```python
from build123d import *

# Parameters (mm, degrees)
ESQUISSE1_R             = 6
BOSS_EXTRU_2_DEPTH      = 10
CONG_2_R                = 1
ESQUISSE5_R             = 4
ENL_V_MAT_EXTRU_2_DEPTH = 14.114877094
COQUE5_T                = -0.2
BOSS_EXTRU_5_REACH      = 14.963


with BuildPart() as part:
    # Esquisse1 → Boss.-Extru.2 (new body)
    with BuildSketch(Plane.XY):
        Circle(ESQUISSE1_R)
    extrude(amount=BOSS_EXTRU_2_DEPTH)

    # Congé2
    cong_2_edges = [part.edges().sort_by_distance(p)[0] for p in [
        (-6, 0, 0),
        (-6, 0, 10),
    ]]
    fillet(cong_2_edges, radius=CONG_2_R)

    # Esquisse5 → Enlèv. mat.-Extru.2 (cut, through all)
    with BuildSketch(Plane.XY.offset(10)):
        Circle(ESQUISSE5_R)
    extrude(amount=-ENL_V_MAT_EXTRU_2_DEPTH, mode=Mode.SUBTRACT)

    # Coque5
    coque5_openings = [part.faces().sort_by_distance(p)[0] for p in [
        (-4, 0, 5),
    ]]
    offset(amount=COQUE5_T, openings=coque5_openings, kind=Kind.INTERSECTION)

    # Esquisse12 → Boss.-Extru.5 (add, up to next)
    with BuildSketch(Plane.XY.offset(0.2), mode=Mode.PRIVATE) as boss_extru_5_sk1:
        with BuildLine():
            ThreePointArc((-4.089017574, 1.521224294), (-4.253433845, 0.970818519), (-4.344112019, 0.403582504))
            ThreePointArc((-4.344112019, 0.403582504), (-4.932642925, 0), (-4.344112019, -0.403582504))
            ThreePointArc((-4.344112019, -0.403582504), (-4.253433845, -0.970818519), (-4.089017574, -1.521224294))
            ThreePointArc((-4.089017574, -1.521224294), (-4.444157712, -2.140193556), (-3.738801802, -2.248454838))
            ThreePointArc((-3.738801802, -2.248454838), (-3.410989107, -2.720173043), (-3.02404305, -3.144733964))
            ThreePointArc((-3.02404305, -3.144733964), (-3.07545256, -3.85649553), (-2.392976034, -3.647993115))
            ThreePointArc((-2.392976034, -3.647993115), (-1.892956143, -3.930763935), (-1.360119712, -4.145390505))
            ThreePointArc((-1.360119712, -4.145390505), (-1.097616311, -4.808971268), (-0.573192015, -4.325001617))
            ThreePointArc((-0.573192015, -4.325001617), (0, -4.362818822), (0.573192015, -4.325001617))
            ThreePointArc((0.573192015, -4.325001617), (1.097616311, -4.808971268), (1.360119712, -4.145390505))
            ThreePointArc((1.360119712, -4.145390505), (1.892956143, -3.930763935), (2.392976034, -3.647993115))
            ThreePointArc((2.392976034, -3.647993115), (3.07545256, -3.85649553), (3.02404305, -3.144733964))
            ThreePointArc((3.02404305, -3.144733964), (3.410989107, -2.720173043), (3.738801802, -2.248454838))
            ThreePointArc((3.738801802, -2.248454838), (4.444157712, -2.140193556), (4.089017574, -1.521224294))
            ThreePointArc((4.089017574, -1.521224294), (4.253433845, -0.970818519), (4.344112019, -0.403582504))
            ThreePointArc((4.344112019, -0.403582504), (4.932642925, 0), (4.344112019, 0.403582504))
            ThreePointArc((4.344112019, 0.403582504), (4.253433845, 0.970818519), (4.089017574, 1.521224294))
            ThreePointArc((4.089017574, 1.521224294), (4.444157712, 2.140193556), (3.738801802, 2.248454838))
            ThreePointArc((3.738801802, 2.248454838), (3.410989107, 2.720173043), (3.02404305, 3.144733964))
            ThreePointArc((3.02404305, 3.144733964), (3.07545256, 3.85649553), (2.392976034, 3.647993115))
            ThreePointArc((2.392976034, 3.647993115), (1.892956143, 3.930763935), (1.360119712, 4.145390505))
            ThreePointArc((1.360119712, 4.145390505), (1.097616311, 4.808971268), (0.573192015, 4.325001617))
            ThreePointArc((0.573192015, 4.325001617), (0, 4.362818822), (-0.573192015, 4.325001617))
            ThreePointArc((-0.573192015, 4.325001617), (-1.097616311, 4.808971268), (-1.360119712, 4.145390505))
            ThreePointArc((-1.360119712, 4.145390505), (-1.892956143, 3.930763935), (-2.392976034, 3.647993115))
            ThreePointArc((-2.392976034, 3.647993115), (-3.07545256, 3.85649553), (-3.02404305, 3.144733964))
            ThreePointArc((-3.02404305, 3.144733964), (-3.410989107, 2.720173043), (-3.738801802, 2.248454838))
            ThreePointArc((-3.738801802, 2.248454838), (-4.444157712, 2.140193556), (-4.089017574, 1.521224294))
        make_face()
        with BuildLine():
            ThreePointArc((-3.940916918, 1.53497163), (-4.123260956, 0.941107406), (-4.216642684, 0.326938116))
            ThreePointArc((-4.216642684, 0.326938116), (-4.067357075, 0), (-4.216642684, -0.326938116))
            ThreePointArc((-4.216642684, -0.326938116), (-4.123260956, -0.941107406), (-3.940916918, -1.53497163))
            ThreePointArc((-3.940916918, -1.53497163), (-3.664562099, -1.764760096), (-3.657210653, -2.124093759))
            ThreePointArc((-3.657210653, -2.124093759), (-3.306598555, -2.636924355), (-2.884644224, -3.092861419))
            ThreePointArc((-2.884644224, -3.092861419), (-2.535955657, -3.179987812), (-2.373423199, -3.500546582))
            ThreePointArc((-2.373423199, -3.500546582), (-1.835023758, -3.810466096), (-1.257032364, -4.038172073))
            ThreePointArc((-1.257032364, -4.038172073), (-0.905072095, -3.965379941), (-0.619550173, -4.183673224))
            ThreePointArc((-0.619550173, -4.183673224), (0, -4.229298294), (0.619550173, -4.183673224))
            ThreePointArc((0.619550173, -4.183673224), (0.905072095, -3.965379941), (1.257032364, -4.038172073))
            ThreePointArc((1.257032364, -4.038172073), (1.835023758, -3.810466096), (2.373423199, -3.500546582))
            ThreePointArc((2.373423199, -3.500546582), (2.535955657, -3.179987812), (2.884644224, -3.092861419))
            ThreePointArc((2.884644224, -3.092861419), (3.306598555, -2.636924355), (3.657210653, -2.124093759))
            ThreePointArc((3.657210653, -2.124093759), (3.664562099, -1.764760096), (3.940916918, -1.53497163))
            ThreePointArc((3.940916918, -1.53497163), (4.123260956, -0.941107406), (4.216642684, -0.326938116))
            ThreePointArc((4.216642684, -0.326938116), (4.067357075, 0), (4.216642684, 0.326938116))
            ThreePointArc((4.216642684, 0.326938116), (4.123260956, 0.941107406), (3.940916918, 1.53497163))
            ThreePointArc((3.940916918, 1.53497163), (3.664562099, 1.764760096), (3.657210653, 2.124093759))
            ThreePointArc((3.657210653, 2.124093759), (3.306598555, 2.636924355), (2.884644224, 3.092861419))
            ThreePointArc((2.884644224, 3.092861419), (2.535955657, 3.179987812), (2.373423199, 3.500546582))
            ThreePointArc((2.373423199, 3.500546582), (1.835023758, 3.810466096), (1.257032364, 4.038172073))
            ThreePointArc((1.257032364, 4.038172073), (0.905072095, 3.965379941), (0.619550173, 4.183673224))
            ThreePointArc((0.619550173, 4.183673224), (0, 4.229298294), (-0.619550173, 4.183673224))
            ThreePointArc((-0.619550173, 4.183673224), (-0.905072095, 3.965379941), (-1.257032364, 4.038172073))
            ThreePointArc((-1.257032364, 4.038172073), (-1.835023758, 3.810466096), (-2.373423199, 3.500546582))
            ThreePointArc((-2.373423199, 3.500546582), (-2.535955657, 3.179987812), (-2.884644224, 3.092861419))
            ThreePointArc((-2.884644224, 3.092861419), (-3.306598555, 2.636924355), (-3.657210653, 2.124093759))
            ThreePointArc((-3.657210653, 2.124093759), (-3.664562099, 1.764760096), (-3.940916918, 1.53497163))
        make_face(mode=Mode.SUBTRACT)
    boss_extru_5_tool1 = extrude(boss_extru_5_sk1.sketch, amount=BOSS_EXTRU_5_REACH, mode=Mode.PRIVATE) - part.part
    add(boss_extru_5_tool1.solids().sort_by_distance((-3.400205, 2.711573, 0.2))[0])


solid = part.part
```
Geometry check sheet. Reference: the model listing, model coordinates, mm. Coordinates: 2 decimals unless noted, no trailing zeros. Answer as a JSON object with one key per item and string values. Group by question number.
Item 1: Depth check by flat-ended pin: pin 1 Ø6.5 at (x, y) = (0, 0) entering from +Z (1 decimal); pin 2 Ø6 at (x, y) = (-2.5, -4.5) entering from -Z; pin 3 Ø5 at (x, z) = (-3.5, 5) entering from +Y; pin 4 Ø1.5 at (x, z) = (-3, 4) entering from +Y. Enter the tip coordinate at first touch or a pass-through.
Item 2: Scan lines: probe 1 along X at (y, z) = (3.25, 4.5); probe 2 along Z at (x, y) = (3.75, 3); probe 3 along Y at (x, z) = (0.75, 4). Record each from-to range of solid material in increasing order.
Item 3: Sectioned sample at A-A, the plane x = 0. Give the number of separate pieces and of enclosed holes in the cut face, and give its area (3 significant figures).
Resolved:
{
 "1": {"pin 1": "through", "pin 2": "z = 0", "pin 3": "y = 5.92", "pin 4": "y = 5.56"},
 "2": {"probe 1": "-5.04 to -4.8, -3.15 to -2.47, 2.47 to 3.15, 4.8 to 5.04", "probe 2": "0 to 0.2, 9.8 to 10", "probe 3": "-5.95 to -5.75, -4.74 to -4.04, 4.04 to 4.74, 5.75 to 5.95"},
 "3": {"separate pieces": "2", "enclosed holes": "2", "area": "7.69 mm^2"}
}
